Part model, mm, in its own coordinate system. A direction names the side the tool comes from. Give positions to 0.01 mm unless a question says otherwise; leave off trailing zeros. Write each loop counter-clockwise with the first axis right and the second up, starting at its lowest first coordinate (ties: lowest second). Pieces come first, ordered by that corner, then holes. Notation, with made-up numbers: M 42,89.25 L 94,89.25 A10 ccw 94,107.25 Z; hole C 0.25,57 d4. An arc over 180 degrees is marked long. Use CSV: the item, a comma, the result in double quotes. Start each with the question number.
1. Band-saw the part on D-D, the plane z = -51. List the corners of the cut face in (x, y), then the cut area to 3 significant figures.
2. Drop flat-ended pins along their axis: pin 1 Ø1 at (y, z) = (106, 48.5) entering from -X; pin 2 Ø10 at (x, y) = (-72, 102.5) entering from -Z; pin 3 Ø5.5 at (y, z) = (70, 0) entering from -X. Give the stop position or say it passes through.
3. Band-saw the part on C-C, the plane x = 88. List the corners of the cut face in (y, z).
4. Band-saw the part on A-A, the plane z = 0. List the corners of the cut face in (x, y), then the cut area to 3 significant figures.
5. Mould opens along Y. For faces 1 (the face through (2, 0, 1)), 2 (the face through (-142, 140, 1)), 3 (the face through (135, 68, 1)), 4 (the face through (-135, 82, -1)) say: pulls with the +Y half, pulls with the -Y half, needs draft (parallel to the pull), parting line crosses it, or undercut.
6. 3-axis set-ups, long thin cutter, end or side, ignore diameter. For faces 5 (the face through (2, 68, -90)), 6 (the face through (137.54, 90.09, 2.2)), 7 (the face through (-2, 64, 95)), 8 (the face through (17.399, 56.285, 92.535)), 9 (the face through (2, 64, -95)): which of +Z, -Z, +X, -X, +Y, -Y reach the whole face in a straight line?
7. Drill centre lines: line 1 along X through (y, z) = (68, 93.5); line 2 along Y through (x, z) = (41.5, -62); line 3 along Z through (x, y) = (-74.5, 119). Where is each one in solid material? Low to high. Write a range as from..to.
8. Band-saw the part on B-B, the plane y = 33.5. List the corners of the cut face in (x, z).
Autodesk Inventor part; units mm, degrees
ref_plane "YZ Plane" through (0, 0, 0) normal (1, 0, 0) x (0, 1, 0)
ref_plane "XZ Plane" through (0, 0, 0) normal (0, 1, 0) x (-1, 0, 0)
ref_plane "XY Plane" through (0, 0, 0) normal (0, 0, 1) x (1, 0, 0)
sketch "Boceto1" plane through (0, 0, 0) normal (0, 1, 0) x (-1, 0, 0)
  line L0 (140, 95) -> (-140, 95)
  line L1 (-140, 95) -> (-140, -95)
  line L2 (-140, -95) -> (140, -95)
  line L3 (140, -95) -> (140, 95)
  point P0 (0, 0)
  dimension "d0" = 280
  dimension "d1" = 190
  dimension "d2" = 95
  dimension "d3" = 140
extrude "Extrusión1" add sketch "Boceto1" along normal blind 130
ref_plane "Plano de trabajo1" through (0, 0, 95) normal (1, 0, 0) x (0, 0, -1)
ref_plane "Plano de trabajo2" through (140, 0, 0) normal (0, 0, -1) x (-1, 0, 0)
sketch "Boceto3" plane through (0, 130, 0) normal (0, 1, 0) x (1, 0, 0)
  line L0 (140, 95) -> (-140, 95)
  line L1 (-140, 95) -> (-140, -95)
  line L2 (-140, -95) -> (140, -95)
  line L3 (140, -95) -> (140, 95)
  line L4 (-135, -90) -> (135, -90)
  line L5 (135, -90) -> (135, 90)
  line L6 (135, 90) -> (-135, 90)
  line L7 (-135, 90) -> (-135, -90)
  point P0 (0, 0)
  dimension "d7" = 270
  dimension "d8" = 135
  dimension "d9" = 180
  dimension "d10" = 90
extrude "Extrusión2" cut sketch "Boceto3" against normal blind 125 contours L7 L6 L5 L4
sketch "Boceto4" plane through (-140, 0, -95) normal (-1, 0, 0) x (0, 0, 1)
  circle A0 centre (95, 29.1709) radius 10
  point P0 (95, 0)
  dimension "d13" = 20
extrude "Extrusión3" [suppressed]
sketch "Boceto7" plane through (-140, 0, 95) normal (0, 0, 1) x (1, 0, 0)
  circle A0 centre (140, 68) radius 10
  line L0 (0, 0) -> (280, 0)
  line L1 (280, 0) -> (280, 130)
  point P0 (140, 0)
  dimension "d18" = 20
  dimension "d19" = 68
  dimension "d20" = 140
extrude "Extrusión5" [suppressed]
sketch "Boceto8" plane through (0, 130, 0) normal (0, 1, 0) x (1, 0, 0)
  line L0 (-142, 97) -> (142, 97)
  line L1 (142, 97) -> (142, -97)
  line L2 (142, -97) -> (-142, -97)
  line L3 (-142, -97) -> (-142, 97)
  line L4 (140, 95) -> (-140, 95)
  line L5 (140, -95) -> (140, 95)
  line L6 (-140, -95) -> (140, -95)
  line L7 (-140, 95) -> (-140, -95)
  point P0 (0, 0)
  dimension "d23" = 2
  dimension "d24" = 2
  dimension "d25" = 2
  dimension "d26" = 2
extrude "Techo" add sketch "Boceto8" along normal blind 20 contours L0 L1 L2 L3 | L5 L6 L7 L4
sketch "Boceto9" plane through (-140, 0, 95) normal (0, 0, 1) x (1, 0, 0)
  circle A0 centre (120, 68) radius 12
  circle A1 centre (160, 68) radius 12
  circle A2 centre (140, 68) radius 10
  line L0 (0, 0) -> (280, 0)
  line L1 (0, 0) -> (0, 130)
  point P0 (140, 0)
  point P1 (148.9, 63.4404)
  point P2 (148.9, 72.5596)
  point P3 (131.1, 63.4404)
  point P4 (131.1, 72.5596)
  dimension "d29" = 24
  dimension "d30" = 24
  dimension "d31" = 68
  dimension "d32" = 40
  dimension "Q" = 120
extrude "Extrusión7" cut sketch "Boceto9" against normal blind 10 contours A0 A2 | A2 A0 | A2 A1 | A1 A2
sketch "Boceto10" plane through (140, 0, 95) normal (1, 0, 0) x (0, 0, -1)
  circle A0 centre (95, 100) radius 10.15
  line L0 (0, 0) -> (0, 130)
  line L1 (0, 130) -> (190, 130)
  point P0 (95, 0)
  dimension "d36" = 20.3
  dimension "d37" = 95
  dimension "d38" = 30
extrude "Extrusión8" cut sketch "Boceto10" against normal blind 10
sketch "Boceto11" plane through (-140, 0, -95) normal (-1, 0, 0) x (0, 0, 1)
  line L0 (0, 130) -> (190, 130)
  circle A0 centre (95, 70) radius 4.5
  line L1 (0, 0) -> (0, 130)
  point P0 (95, 0)
  dimension "d45" = 9
  dimension "d46" = 60
  dimension "d47" = 95
extrude "Extrusión10" cut sketch "Boceto11" against normal blind 10
properties part number "cajaEléctrica"
Output:
1,outline,"M -142,130 L -140,130 L -140,0 L 140,0 L 140,130 L 142,130 L 142,150 L -142,150 Z; hole M -135,5 L 135,5 L 135,130 L -135,130 Z"
1,area,"8,330 mm²"
2,pin 1,"stops at x = -140"
2,pin 2,"stops at z = -95"
2,pin 3,"stops at x = 135"
3,outline,"M 0,-95 L 130,-95 L 130,-97 L 150,-97 L 150,97 L 130,97 L 130,95 L 0,95 Z; hole M 5,-90 L 130,-90 L 130,90 L 5,90 Z"
4,outline,"M -142,130 L -140,130 L -140,74.5 L -135,74.5 L -135,130 L 135,130 L 135,110.15 L 140,110.15 L 140,130 L 142,130 L 142,150 L -142,150 Z; M -140,0 L 140,0 L 140,89.85 L 135,89.85 L 135,5 L -135,5 L -135,65.5 L -140,65.5 Z"
4,area,"8,180 mm²"
5,face 1,"pulls with the -Y half"
5,face 2,"needs draft"
5,face 3,"undercut"
5,face 4,"undercut"
6,face 5,"none"
6,face 6,"+X"
6,face 7,"+Z, +X, -X, -Y"
6,face 8,"+Z"
6,face 9,"-Z, +X, -X, -Y"
7,line 1,"x = -140..-32, -8..8, 32..140"
7,line 2,"y = 0..5, 130..150"
7,line 3,"z = -95..-90, 90..95"
8,outline,"M -140,-95 L 140,-95 L 140,95 L -140,95 Z; hole M -135,-90 L 135,-90 L 135,90 L -135,90 Z"
